Check sheet for the modelled part. Datum: model origin and axes. Units: mm. Give positions to 0.01 mm unless a question says otherwise; leave off trailing zeros. Order: outer loops, then holes, each group sorted by start corner. A loop starts at its lowest first (then second) coordinate and runs counter-clockwise, first axis right, second up.
from build123d import *

# Parameters (mm, degrees)
SKETCH_1_W      = 29
SKETCH_1_H      = 12.7
EXTRUDE_1_DEPTH = 15.7
EXTRUDE_2_DEPTH = 3.5
FILLET_1_R      = 0.05
CHAMFER_1_SIZE  = 1.5
FILLET_2_R      = 0.75


with BuildPart() as part:
    # Эскиз1 → Бобышка-Вытянуть1 (new body)
    with BuildSketch(Plane(origin=(0, 0, 0), x_dir=(1, 0, 0), z_dir=(0, 1, 0))):
        Rectangle(SKETCH_1_W, SKETCH_1_H)
    extrude(amount=EXTRUDE_1_DEPTH)

    # Эскиз2 → Бобышка-Вытянуть2 (add)
    with BuildSketch(Plane.XZ):
        with BuildLine():
            Line((-12.3, 4.15), (-11.9, 4.15))
            ThreePointArc((-11.9, 4.15), (-11.864644661, 4.135355339), (-11.85, 4.1))
            Line((-11.85, 4.1), (-11.85, 3.4))
            ThreePointArc((-11.85, 3.4), (-11.864644661, 3.364644661), (-11.9, 3.35))
            Line((-11.9, 3.35), (-12.3, 3.35))
            ThreePointArc((-12.3, 3.35), (-12.335355339, 3.364644661), (-12.35, 3.4))
            Line((-12.35, 3.4), (-12.35, 4.1))
            ThreePointArc((-12.35, 4.1), (-12.335355339, 4.135355339), (-12.3, 4.15))
        make_face()
        with BuildLine():
            Line((7.65, 4.1), (7.65, 3.4))
            ThreePointArc((7.65, 3.4), (7.664644661, 3.364644661), (7.7, 3.35))
            Line((7.7, 3.35), (8.1, 3.35))
            ThreePointArc((8.1, 3.35), (8.135355339, 3.364644661), (8.15, 3.4))
            Line((8.15, 3.4), (8.15, 4.1))
            ThreePointArc((8.15, 4.1), (8.135355339, 4.135355339), (8.1, 4.15))
            Line((8.1, 4.15), (7.7, 4.15))
            ThreePointArc((7.7, 4.15), (7.664644661, 4.135355339), (7.65, 4.1))
        make_face()
        with BuildLine():
            Line((12.65, 4.1), (12.65, 3.4))
            ThreePointArc((12.65, 3.4), (12.664644661, 3.364644661), (12.7, 3.35))
            Line((12.7, 3.35), (13.1, 3.35))
            ThreePointArc((13.1, 3.35), (13.135355339, 3.364644661), (13.15, 3.4))
            Line((13.15, 3.4), (13.15, 4.1))
            ThreePointArc((13.15, 4.1), (13.135355339, 4.135355339), (13.1, 4.15))
            Line((13.1, 4.15), (12.7, 4.15))
            ThreePointArc((12.7, 4.15), (12.664644661, 4.135355339), (12.65, 4.1))
        make_face()
        with BuildLine():
            Line((7.65, -3.4), (7.65, -4.1))
            ThreePointArc((7.65, -4.1), (7.664644661, -4.135355339), (7.7, -4.15))
            Line((7.7, -4.15), (8.1, -4.15))
            ThreePointArc((8.1, -4.15), (8.135355339, -4.135355339), (8.15, -4.1))
            Line((8.15, -4.1), (8.15, -3.4))
            ThreePointArc((8.15, -3.4), (8.135355339, -3.364644661), (8.1, -3.35))
            Line((8.1, -3.35), (7.7, -3.35))
            ThreePointArc((7.7, -3.35), (7.664644661, -3.364644661), (7.65, -3.4))
        make_face()
        with BuildLine():
            Line((12.65, -3.4), (12.65, -4.1))
            ThreePointArc((12.65, -4.1), (12.664644661, -4.135355339), (12.7, -4.15))
            Line((12.7, -4.15), (13.1, -4.15))
            ThreePointArc((13.1, -4.15), (13.135355339, -4.135355339), (13.15, -4.1))
            Line((13.15, -4.1), (13.15, -3.4))
            ThreePointArc((13.15, -3.4), (13.135355339, -3.364644661), (13.1, -3.35))
            Line((13.1, -3.35), (12.7, -3.35))
            ThreePointArc((12.7, -3.35), (12.664644661, -3.364644661), (12.65, -3.4))
        make_face()
        with BuildLine():
            Line((-12.35, -3.4), (-12.35, -4.1))
            ThreePointArc((-12.35, -4.1), (-12.335355339, -4.135355339), (-12.3, -4.15))
            Line((-12.3, -4.15), (-11.9, -4.15))
            ThreePointArc((-11.9, -4.15), (-11.864644661, -4.135355339), (-11.85, -4.1))
            Line((-11.85, -4.1), (-11.85, -3.4))
            ThreePointArc((-11.85, -3.4), (-11.864644661, -3.364644661), (-11.9, -3.35))
            Line((-11.9, -3.35), (-12.3, -3.35))
            ThreePointArc((-12.3, -3.35), (-12.335355339, -3.364644661), (-12.35, -3.4))
        make_face()
    extrude(amount=EXTRUDE_2_DEPTH)

    # Скругление1
    fillet_1_edges = [part.edges().sort_by_distance(p)[0] for p in [
        (12.664644661, -3.5, -4.135355339),
        (12.9, -3.5, -4.15),
        (13.135355339, -3.5, -4.135355339),
        (13.15, -3.5, -3.75),
        (13.135355339, -3.5, -3.364644661),
        (12.9, -3.5, -3.35),
        (12.664644661, -3.5, -3.364644661),
        (12.65, -3.5, -3.75),
        (-12.335355339, -3.5, -4.135355339),
        (-12.1, -3.5, -4.15),
        (-11.864644661, -3.5, -4.135355339),
        (-11.85, -3.5, -3.75),
        (-11.864644661, -3.5, -3.364644661),
        (-12.1, -3.5, -3.35),
        (-12.335355339, -3.5, -3.364644661),
        (-12.35, -3.5, -3.75),
        (-12.335355339, -3.5, 3.364644661),
        (-12.1, -3.5, 3.35),
        (-11.864644661, -3.5, 3.364644661),
        (-11.85, -3.5, 3.75),
        (-11.864644661, -3.5, 4.135355339),
        (-12.1, -3.5, 4.15),
        (-12.335355339, -3.5, 4.135355339),
        (-12.35, -3.5, 3.75),
        (7.664644661, -3.5, 3.364644661),
        (7.9, -3.5, 3.35),
        (8.135355339, -3.5, 3.364644661),
        (8.15, -3.5, 3.75),
        (8.135355339, -3.5, 4.135355339),
        (7.9, -3.5, 4.15),
        (7.664644661, -3.5, 4.135355339),
        (7.65, -3.5, 3.75),
        (12.664644661, -3.5, 3.364644661),
        (12.9, -3.5, 3.35),
        (13.135355339, -3.5, 3.364644661),
        (13.15, -3.5, 3.75),
        (13.135355339, -3.5, 4.135355339),
        (12.9, -3.5, 4.15),
        (12.664644661, -3.5, 4.135355339),
        (12.65, -3.5, 3.75),
        (7.664644661, -3.5, -4.135355339),
        (7.9, -3.5, -4.15),
        (8.135355339, -3.5, -4.135355339),
        (8.15, -3.5, -3.75),
        (8.135355339, -3.5, -3.364644661),
        (7.9, -3.5, -3.35),
        (7.664644661, -3.5, -3.364644661),
        (7.65, -3.5, -3.75),
    ]]
    fillet(fillet_1_edges, radius=FILLET_1_R)

    # Фаска1
    chamfer_1_edges = [part.edges().sort_by_distance(p)[0] for p in [
        (14.5, 15.7, 0),
    ]]
    chamfer(chamfer_1_edges, length=CHAMFER_1_SIZE)

    # Скругление2
    fillet_2_edges = [part.edges().sort_by_distance(p)[0] for p in [
        (-14.5, 15.7, 0),
        (-0.75, 15.7, 6.35),
        (-0.75, 15.7, -6.35),
        (13, 15.7, 0),
        (14.5, 7.1, -6.35),
        (13.75, 14.95, -6.35),
        (14.5, 7.1, 6.35),
        (14.5, 14.2, 0),
        (13.75, 14.95, 6.35),
        (-14.5, 7.85, 6.35),
        (-14.5, 7.85, -6.35),
    ]]
    fillet(fillet_2_edges, radius=FILLET_2_R)


solid = part.part
1) Section check A-A, the plane z = -2. Record the cut outline in (x, y), then the cut area to 3 significant figures.
Recorded:
outline: (-14.5, 0) - (14.5, 0) - (14.5, 13.89) arc R0.75 ccw to (14.28, 14.42) - (13.22, 15.48) arc R0.75 ccw to (12.69, 15.7) - (-13.75, 15.7) arc R0.75 ccw to (-14.5, 14.95) - close
area: 454 mm2
2) Material ranges on L1, parallel to Y at x = 7.75, z = 0; L2, parallel to Y at x = -10.5, z = 6; L3, parallel to X at y = 14.25, z = 1.5, recorded low to high.
Recorded:
L1: y = 0 to 15.7
L2: y = 0 to 15.58
L3: x = -14.5 to 14.41
3) Section check D-D, the plane z = -3.75. Record the cut outline in (x, y).
Recorded:
outline: (-14.5, 0) - (-12.35, 0) - (-12.35, -3.45) arc R0.05 ccw to (-12.3, -3.5) - (-11.9, -3.5) arc R0.05 ccw to (-11.85, -3.45) - (-11.85, 0) - (7.65, 0) - (7.65, -3.45) arc R0.05 ccw to (7.7, -3.5) - (8.1, -3.5) arc R0.05 ccw to (8.15, -3.45) - (8.15, 0) - (12.65, 0) - (12.65, -3.45) arc R0.05 ccw to (12.7, -3.5) - (13.1, -3.5) arc R0.05 ccw to (13.15, -3.45) - (13.15, 0) - (14.5, 0) - (14.5, 13.89) arc R0.75 ccw to (14.28, 14.42) - (13.22, 15.48) arc R0.75 ccw to (12.69, 15.7) - (-13.75, 15.7) arc R0.75 ccw to (-14.5, 14.95) - close
4) Section check B-B, the plane x = 5.75. Record the cut outline in (y, z), then the cut area to 3 significant figures.
Recorded:
outline: (0, -6.35) - (14.95, -6.35) arc R0.75 ccw to (15.7, -5.6) - (15.7, 5.6) arc R0.75 ccw to (14.95, 6.35) - (0, 6.35) - close
area: 199 mm2
5) Section check C-C, the plane y = -1.25. State how many separate pieces and enclosed holes the cut face has, then the cut area to 3 significant figures.
Recorded:
separate pieces: 6
enclosed holes: 0
area: 2.39 mm2
6) Depth check by flat-ended pin: pin 1 Ø0.8 at (y, z) = (-1, -4) entering from -X; pin 2 Ø5 at (x, z) = (-0.5, 1.5) entering from -Y; pin 3 Ø1 at (y, z) = (-1, -1) entering from -X; pin 4 Ø0.6 at (y, z) = (-1, -3.5) entering from +X. Enter the tip coordinate at first touch or a pass-through.
Recorded:
pin 1: stops at x = -12.35
pin 2: stops at y = 0
pin 3: passes through
pin 4: stops at x = 13.15
